For this review, take the finished solid that the model builds, in its own axes (mm). Face numbers are marked on the shaded views. Round coordinates to 2 decimals unless told otherwise and drop trailing zeros. Write each loop counter-clockwise with the first axis right and the second up, starting at its lowest first coordinate (ties: lowest second). Pieces come first, ordered by that corner, then holes. Notation, with made-up numbers: (16.25, -30) - (29.25, -30) arc R22 ccw to (29.25, 1) - close; hole circle Ø3 at (89, 20). An arc over 180 degrees is marked (long way). One line per item, written item: value. Start each with the question number.
Q1. Mouldability with a two-part tool opening along Z and no side actions: class the marked faces 1, 2 and 3 as +Z half, -Z half, draft (parallel to the pull), parting line (faces both ways), or undercut.
Q2. Add section C-C on z = 31.5. Write out the cut boundary in (x, y).
Q3. Add section D-D on z = 44.5. Write out the cut boundary in (x, y).
Q4. Clearance check with flat-ended pins moving along their axes: pin 1 Ø8 at (y, z) = (10.5, 32) entering from +X; pin 2 Ø6 at (x, z) = (15.5, 36) entering from -Y; pin 3 Ø1.5 at (x, z) = (0, 37.5) entering from +Y. State where each tip first meets the part, or that it passes through.
Q5. Add section A-A on y = 0. Write out the cut boundary in (x, z).
Q6. For probe 1 along Y at (x, z) = (0, 4.75); probe 2 along Z at (x, y) = (2, 3.5); probe 3 along Y at (x, z) = (-6, 18.5), list the stretches that pass through material, from the lowest coordinate up.
```python
from build123d import *

# Parameters (mm, degrees)
F0_R     = 17.5339973563
F1_DEPTH = 50.8
F2_R     = 24.353495683
F3_DEPTH = 7.874
F5_T     = -7.62


# Not quite as in the source:
# - a fillet or chamfer that OpenCascade refuses, or shapes differently, is made with other operations: its cross-section is extruded or revolved along the edge and cut away or added


with BuildPart() as f1:
    # F0 (on Top) → F1 (new body)
    with BuildSketch(Plane.XY):
        Circle(F0_R)
    extrude(amount=F1_DEPTH)

    # F2 (on Top) → F3 (join)
    with BuildSketch(Plane.XY):
        Circle(F2_R)
    extrude(amount=F3_DEPTH)

    # F4: fillet of radius 120.1892079892 on 1 edges, made by hand

    # F4_s1 → F4_t2 (revolve)
    with BuildSketch(Plane.XZ):
        with BuildLine():
            ThreePointArc((24.353495683, 7.874), (19.2511383183, 27.5394411034), (17.5339973563, 47.7833303391))
            Line((17.5339973563, 47.7833303391), (17.5339973563, 7.874))
            Line((17.5339973563, 7.874), (24.353495683, 7.874))
        make_face()
    revolve(axis=Axis((0, 0, 7.874), (0, 0, -1)))

    # F5
    f5_openings = [f1.faces().sort_by_distance(p)[0] for p in [
        (0, 0, 0),
    ]]
    offset(amount=F5_T, openings=f5_openings)


solid = f1.part
```
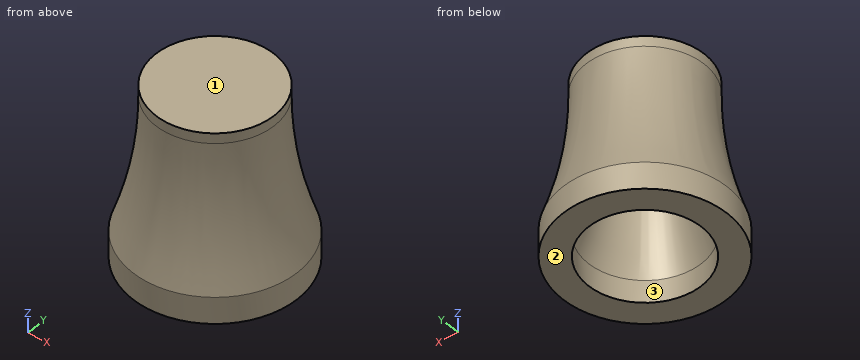
Result set:
1. face 1: +Z half
1. face 2: -Z half
1. face 3: draft
2. outline: circle Ø37.28 at (0, 0); hole circle Ø21.91 at (0, 0)
3. outline: circle Ø35.16 at (0, 0)
4. pin 1: stops at x = 17.51
4. pin 2: stops at y = -13.14
4. pin 3: stops at y = 18.04
5. outline: (-24.35, 0) - (-16.73, 0) - (-16.73, 6.59) arc R127.81 ccw to (-10, 43.18) - (10, 43.18) arc R127.81 ccw to (16.73, 6.59) - (16.73, 0) - (24.35, 0) - (24.35, 7.87) arc R120.19 cw to (17.53, 47.78) - (17.53, 50.8) - (-17.53, 50.8) - (-17.53, 47.78) arc R120.19 cw to (-24.35, 7.87) - close
6. probe 1: y = -24.35 to -16.73, 16.73 to 24.35
6. probe 2: z = 43.18 to 50.8
6. probe 3: y = -20.29 to -11.89, 11.89 to 20.29
